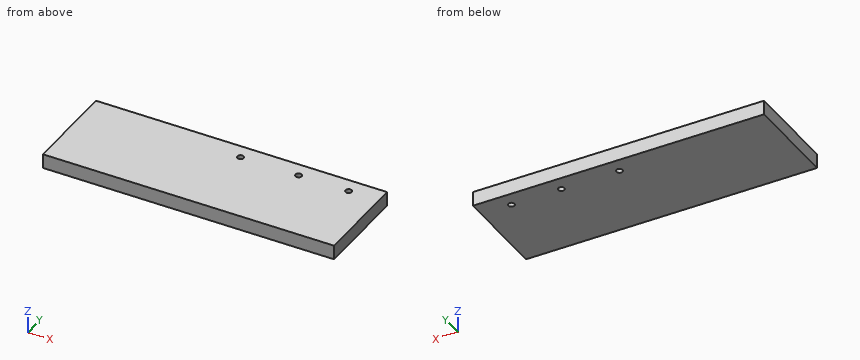
Autodesk Inventor part; units mm, degrees
ref_plane "YZ Plane" through (0, 0, 0) normal (1, 0, 0) x (0, 1, 0)
ref_plane "XZ Plane" through (0, 0, 0) normal (0, 1, 0) x (-1, 0, 0)
ref_plane "XY Plane" through (0, 0, 0) normal (0, 0, 1) x (1, 0, 0)
sketch "Sketch1" plane through (0, 0, 0) normal (0, 0, 1) x (1, 0, 0)
  line L0 (0, 0) -> (369.57, 0)
  line L1 (369.57, 0) -> (369.57, -120.65)
  line L2 (369.57, -120.65) -> (0, -120.65)
  line L3 (0, -120.65) -> (0, 0)
  circle A0 centre (331.47, -19.05) radius 3.9179
  circle A1 centre (267.97, -19.05) radius 3.9243
  circle A2 centre (194.31, -19.05) radius 3.9243
  dimension "d0" = 369.57
  dimension "d1" = 120.65
  dimension "d2" = 7.8359
  dimension "d3" = 38.1
  dimension "d4" = 101.6
  dimension "d5" = 7.8486
  dimension "d6" = 101.6
  dimension "d7" = 63.5
  dimension "d8" = 7.8486
  dimension "d9" = 101.6
  dimension "d10" = 73.66
extrude "Extrusion1" add sketch "Sketch1" against normal blind 18.3261
properties part number "Kermit bumper Medium"
Here's how the part is built. I have some questions about the finished solid (model axes, mm). Coordinates: 2 decimals unless noted, no trailing zeros. Order: outer loops, then holes, each group sorted by start corner. A loop starts at its lowest first (then second) coordinate and runs counter-clockwise, first axis right, second up.
1) Will these pins go through, and if not, where does the flat tip stop? pin 1 (10 mm diameter, centred on x = 194.31, y = -19.05, fed in from +Z); pin 2 (7 mm diameter, centred on x = 331.47, y = -19.05, fed in from -Z).
2) I need wall thicknesses on line 1 (X direction, y = -19, z = -11.25); line 2 (Y direction, x = 331, z = -2.25); line 3 (Y direction, x = 194.31, z = -6.5). Which ranges of each line are inside material? Lowest first, please.
3) Imagine slicing it at B-B on y = -19.05. List the corners of the cut face in (x, z) for me, and give its area (3 significant figures).
4) Imagine slicing it at A-A on x = 331.47. List the corners of the cut face in (y, z) for me, and give its area (3 significant figures).
Response values:
1. pin 1: stops at z = 0
1. pin 2: passes through
2. line 1: x = 0 to 190.39, 198.23 to 264.05, 271.89 to 327.55, 335.39 to 369.57
2. line 2: y = -120.65 to -22.94, -15.16 to 0
2. line 3: y = -120.65 to -22.97, -15.13 to 0
3. outline: (0, -18.33) - (190.39, -18.33) - (190.39, 0) - (0, 0) - close; (198.23, -18.33) - (264.05, -18.33) - (264.05, 0) - (198.23, 0) - close; (271.89, -18.33) - (327.55, -18.33) - (327.55, 0) - (271.89, 0) - close; (335.39, -18.33) - (369.57, -18.33) - (369.57, 0) - (335.39, 0) - close
3. area: 6,340 mm2
4. outline: (-120.65, -18.33) - (-22.97, -18.33) - (-22.97, 0) - (-120.65, 0) - close; (-15.13, -18.33) - (0, -18.33) - (0, 0) - (-15.13, 0) - close
4. area: 2,070 mm2
